Here's how the part is built. I have some questions about the finished solid (model axes, mm). A direction names the side the tool comes from. Round coordinates to 2 decimals unless told otherwise and drop trailing zeros. Write each loop counter-clockwise with the first axis right and the second up, starting at its lowest first coordinate (ties: lowest second). Pieces come first, ordered by that corner, then holes. Notation, with made-up numbers: (-11.75, -30) -> (17.25, -30) arc R22 cw to (17.25, -11) -> close; hole circle Ø4 at (-35.5, -12). An arc over 180 degrees is marked (long way). Put each result on its own line as item: value. Start each with the question number.
1. For pin 1 (1 mm diameter, centred on x = -49.5, z = 40, fed in from -Y); pin 2 (3 mm diameter, centred on x = -39.5, z = 54.5, fed in from +Y), each with a flat end and sliding along its axis, tell me the tip position at first contact or that it passes through.
2. We'd pull the mould along Z, two halves only. Please class faces 1 (the face through (-50, 0, 59.832)), 2 (the face through (-50, -14, 31.301)), 3 (the face through (-50, 0, 28.801)), 4 (the face through (-75.622, 0, 44)): +Z half, -Z half, draft (parallel to the pull), parting line (faces both ways), or undercut.
3. Which directions (+Z, -Z, +X, -X, +Y, -Y) give clear straight access to the entire face, cutting with the end or side of a thin tool? Please do faces 5 (the face through (-50, -14, 57.332)), 6 (the face through (-50, 2.5, 44)), 7 (the face through (-24.342, 0, 44)).
4. I need wall thicknesses on probe 1 along X at (y, z) = (-15.5, 35.5); probe 2 along Z at (x, y) = (-68.5, 12); probe 3 along Y at (x, z) = (-34.5, 43.5). Which ranges of each line are inside material? Lowest first, please. Write a range as from..to.
5. Suppose I cut it at C-C (z = 42). Please give me the cut outline in (x, y).
6. Suppose I cut it at A-A (y = -9). Please give me the cut outline in (x, z), then the cut area to 3 significant figures.
7. Suppose I cut it at B-B (x = -60.5). Please give me the cut outline in (y, z), then the cut area to 3 significant figures.
```python
from build123d import *

# Parameters (mm, degrees)
F0_W     = 51.280171
F0_H     = 31.031217
F1_DEPTH = 25
F2_T     = -2.5


with BuildPart() as f1:
    # F0 (on Front) → F1 (new body)
    with BuildSketch(Plane.XZ):
        with Locations((-49.981937, 44.316455)):
            Rectangle(F0_W, F0_H)
    extrude(amount=F1_DEPTH)

    # F2
    f2_openings = [f1.faces().sort_by_distance(p)[0] for p in [
        (-49.981937, -25, 44.316456),
    ]]
    offset(amount=F2_T, openings=f2_openings)

    # F3: F1 across face


with BuildPart() as f1_1:
    add(f1.part)
    add(f1.part.mirror(Plane(origin=(-49.981937, 0, 44.316456), x_dir=(1, 0, 0), z_dir=(0, 1, 0))))


solid = f1_1.part
```
Verdict:
1. pin 1: stops at y = -2.5
1. pin 2: stops at y = 2.5
2. face 1: +Z half
2. face 2: undercut
2. face 3: -Z half
2. face 4: draft
3. face 5: -Y
3. face 6: +Y
3. face 7: +Z, -Z, +X, +Y, -Y
4. probe 1: x = -75.62..-73.12, -26.84..-24.34
4. probe 2: z = 28.8..31.3, 57.33..59.83
4. probe 3: y = -2.5..2.5
5. outline: (-75.62, -25) -> (-73.12, -25) -> (-73.12, -2.5) -> (-26.84, -2.5) -> (-26.84, -25) -> (-24.34, -25) -> (-24.34, 25) -> (-26.84, 25) -> (-26.84, 2.5) -> (-73.12, 2.5) -> (-73.12, 25) -> (-75.62, 25) -> close
6. outline: (-75.62, 28.8) -> (-24.34, 28.8) -> (-24.34, 59.83) -> (-75.62, 59.83) -> close; hole (-73.12, 31.3) -> (-26.84, 31.3) -> (-26.84, 57.33) -> (-73.12, 57.33) -> close
6. area: 387 mm^2
7. outline: (-25, 28.8) -> (25, 28.8) -> (25, 31.3) -> (2.5, 31.3) -> (2.5, 57.33) -> (25, 57.33) -> (25, 59.83) -> (-25, 59.83) -> (-25, 57.33) -> (-2.5, 57.33) -> (-2.5, 31.3) -> (-25, 31.3) -> close
7. area: 380 mm^2
